```python
from build123d import *

# Parameters (mm, degrees)
SKETCH1_R           = 3.175
BOSS_EXTRUDE1_DEPTH = 6.096
CUT_EXTRUDE1_DEPTH  = 8.636
SKETCH4_W           = 6.096
SKETCH4_H           = 7.62
CUT_EXTRUDE2_DEPTH  = 81.243500547
SKETCH5_R           = 1.651
CUT_EXTRUDE4_DEPTH  = 6.096
CUT_EXTRUDE5_DEPTH  = 6.096


with BuildPart() as part:
    # Sketch1 → Boss-Extrude1 (new body)
    with BuildSketch(Plane.XY):
        Polygon((0, 0), (-38.1, 0), (-38.1, -7.62), (-32.004, -7.62), (-32.004, -15.24), (-38.1, -15.24), (-38.1, -22.86), (-32.004, -22.86), (-32.004, -30.48), (-38.1, -30.48), (-38.1, -38.1), (-32.004, -38.1), (-32.004, -45.72), (-38.1, -45.72), (-38.1, -70.358), (0, -50.8), align=None)
        with Locations(Location((-8.382, -8.382, 0), (0, 0, 180))):
            Circle(SKETCH1_R, mode=Mode.SUBTRACT)
    extrude(amount=BOSS_EXTRUDE1_DEPTH)

    # Sketch2 → Cut-Extrude1 (cut)
    with BuildSketch(Plane(origin=(0, 0, 0), x_dir=(-1, 0, 0), z_dir=(0, 0, -1))):
        Polygon((38.1, 0), (12.7, 0), (38.1, -3.81), align=None)
    extrude(amount=-CUT_EXTRUDE1_DEPTH, mode=Mode.SUBTRACT)

    # Sketch4 → Cut-Extrude2 (cut, through all)
    with BuildSketch(Plane.XY.offset(6.096)):
        with Locations((-35.052, -57.15)):
            Rectangle(SKETCH4_W, SKETCH4_H)
    extrude(amount=-CUT_EXTRUDE2_DEPTH, mode=Mode.SUBTRACT)

    # Sketch5 → Cut-Extrude4 (cut)
    with BuildSketch(Plane(origin=(0, 0, 0), x_dir=(-1, 0, 0), z_dir=(0, 0, -1))):
        with Locations((10.982204311, -29.558964691)):
            Circle(SKETCH5_R)
    extrude(amount=-CUT_EXTRUDE4_DEPTH, mode=Mode.SUBTRACT)

    # Sketch6 → Cut-Extrude5 (cut)
    with BuildSketch(Plane.XY.offset(6.096)):
        Polygon((-5.230665969, -8.768935165), (-4.600399162, -8.846322198), (-7.200603473, -30.02328689), (-9.343510615, -29.760170977), (-12.620898007, -29.357758405), (-14.763805149, -29.094642493), (-12.163600838, -7.917677802), (-11.533334031, -7.995064835), align=None)
    extrude(amount=-CUT_EXTRUDE5_DEPTH, mode=Mode.SUBTRACT)


solid = part.part
```
Design review of the part built by this model. Coordinates are the model's own, in mm. A direction names the side the tool comes from. Give positions to 0.01 mm unless a question says otherwise; leave off trailing zeros. Order: outer loops, then holes, each group sorted by start corner. A loop starts at its lowest first (then second) coordinate and runs counter-clockwise, first axis right, second up. Notation, with made-up numbers: (-31, -22) - (-2, -22) arc R18 cw to (-2, -3) - close; hole circle Ø7 at (37.25, 9). An arc over 180 degrees is marked (long way). Use a Markdown table: item, result. Add a question column.
(1) Add section B-B on x = -10.5. Give the boundary of the cut face in (y, z), then the cut area to 3 significant figures.
(2) Wall thickness on probe 1 along Y at (x, z) = (-34.5, 3.5); probe 2 along X at (y, z) = (-43.5, 3.5); probe 3 along X at (y, z) = (-18.5, 4.5): over which ranges is each line inside the solid? List them lowest first. Write a range as [from, to].
(3) Machinability: for faces 4 (the face through (-11.15, -31.2, 3.01)), 5 (the face through (-6, 0, 3)), 6 (the face through (-35, -45.72, 3)), which of the approach directions +Z, -Z, +X, -X, +Y, -Y give a long, thin tool a straight path to every point of the face, cutting with its end or side? Answer none if there is none.
(4) Mouldability with a two-part tool opening along Y and no side actions: class faces 1 (the face through (-35, -53.34, 3)), 2 (the face through (-19, -35, 6.096)), 3 (the face through (-19.317, -60.716, 3.005)) as +Y half, -Y half, draft (parallel to the pull), parting line (faces both ways), or undercut.
(5) Clearance check with flat-ended pins moving along their axes: P1, Ø3, axis at x = -36, z = 2, coming from the -Y side; P2, Ø1.5, axis at x = -19.5, z = 3, coming from the +Y side; P3, Ø2, axis at x = -18.5, z = 4, coming from the -Y side. State where each tip first meets the part, or that it passes through.
(6) Add section C-C on y = -18. Give the boundary of the cut face in (x, z), then the cut area to 3 significant figures.
(7) Add section D-D on x = -36. Give the boundary of the cut face in (y, z) (3 decimals), then the cut area to 3 significant figures.
Report:
| question | item | result |
|---|---|---|
| 1 | outline | (-56.19, 0) - (-31.14, 0) - (-31.14, 6.1) - (-56.19, 6.1) - close; (-6.02, 0) - (0, 0) - (0, 6.1) - (-6.02, 6.1) - close |
| 1 | area | 189 mm² |
| 2 | probe 1 | y = [-68.51, -60.96], [-53.34, -45.72], [-38.1, -30.48], [-22.86, -15.24], [-7.62, -3.27] |
| 2 | probe 2 | x = [-32, 0] |
| 2 | probe 3 | x = [-38.1, -13.46], [-5.79, 0] |
| 3 | face 4 | +Z, -Z |
| 3 | face 5 | +Z, -Z, +X, -X, +Y |
| 3 | face 6 | +Z, -Z, -X |
| 4 | face 1 | undercut |
| 4 | face 2 | draft |
| 4 | face 3 | -Y half |
| 5 | P1 | stops at y = -70.05 |
| 5 | P2 | stops at y = -0.91 |
| 5 | P3 | stops at y = -60.81 |
| 6 | outline | (-38.1, 0) - (-13.4, 0) - (-13.4, 6.1) - (-38.1, 6.1) - close; (-5.72, 0) - (0, 0) - (0, 6.1) - (-5.72, 6.1) - close |
| 6 | area | 185 mm² |
| 7 | outline | (-69.28, 0) - (-60.96, 0) - (-60.96, 6.096) - (-69.28, 6.096) - close; (-53.34, 0) - (-45.72, 0) - (-45.72, 6.096) - (-53.34, 6.096) - close; (-38.1, 0) - (-30.48, 0) - (-30.48, 6.096) - (-38.1, 6.096) - close; (-22.86, 0) - (-15.24, 0) - (-15.24, 6.096) - (-22.86, 6.096) - close; (-7.62, 0) - (-3.495, 0) - (-3.495, 6.096) - (-7.62, 6.096) - close |
| 7 | area | 215 mm² |
